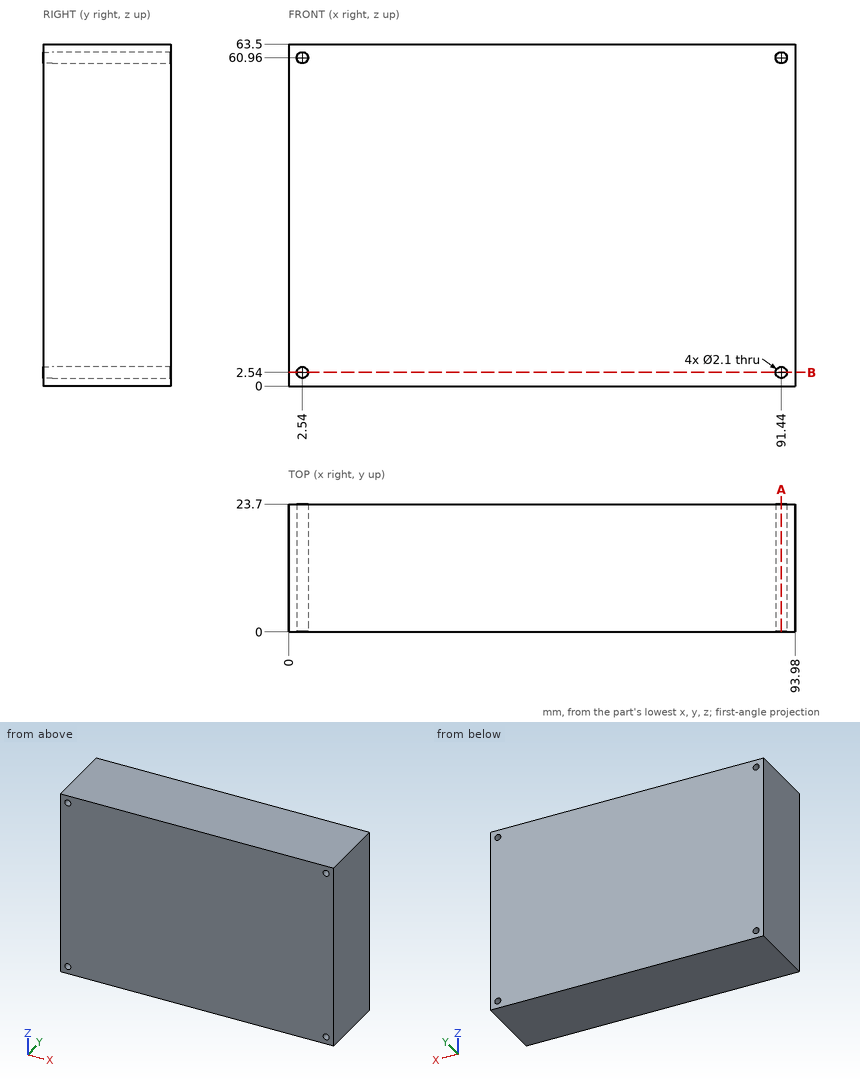
Drawing for the job (mm, zero at the part's lowest x, y, z). Round coordinates to 2 decimals unless told otherwise and drop trailing zeros. Write each loop counter-clockwise with the first axis right and the second up, starting at its lowest first coordinate (ties: lowest second). Pieces come first, ordered by that corner, then holes. Notation, with made-up numbers: (57.5, 54.25) - (93.5, 54.25) arc R28 ccw to (93.5, 78.25) - close; hole circle Ø3 at (-28, 36.5). An arc over 180 degrees is marked (long way). Return JSON: item names as keys, results as strings. Group by question number.
Item 1: Band-saw the part on A-A on x = 91.44. List the corners of the cut face in (y, z), plus the area to 3 significant figures.
Item 2: Probe probe 1 along X at (y, z) = (8.5, 60.96); probe 2 along Z at (x, y) = (91.44, 15). List the from-to ranges inside material, lowest first.
Item 3: Band-saw the part on B-B on z = 2.54. List the corners of the cut face in (x, y).
Item 4: Flat gauge pin, fed straight in: pin 1 Ø1.3 at (x, z) = (91.44, 2.54) entering from +Y. Where does the tip first touch, or does it go through?
Resolved:
{
 "1": {"outline": "(0, 0) - (23.7, 0) - (23.7, 1.49) - (0, 1.49) - close; (0, 3.59) - (23.7, 3.59) - (23.7, 59.91) - (0, 59.91) - close; (0, 62.01) - (23.7, 62.01) - (23.7, 63.5) - (0, 63.5) - close", "area": "1,410 mm²"},
 "2": {"probe 1": "x = 0 to 1.49, 3.59 to 90.39, 92.49 to 93.98", "probe 2": "z = 0 to 1.49, 3.59 to 59.91, 62.01 to 63.5"},
 "3": {"outline": "(0, 0) - (1.49, 0) - (1.49, 23.7) - (0, 23.7) - close; (3.59, 0) - (90.39, 0) - (90.39, 23.7) - (3.59, 23.7) - close; (92.49, 0) - (93.98, 0) - (93.98, 23.7) - (92.49, 23.7) - close"},
 "4": {"pin 1": "passes through"}
}
